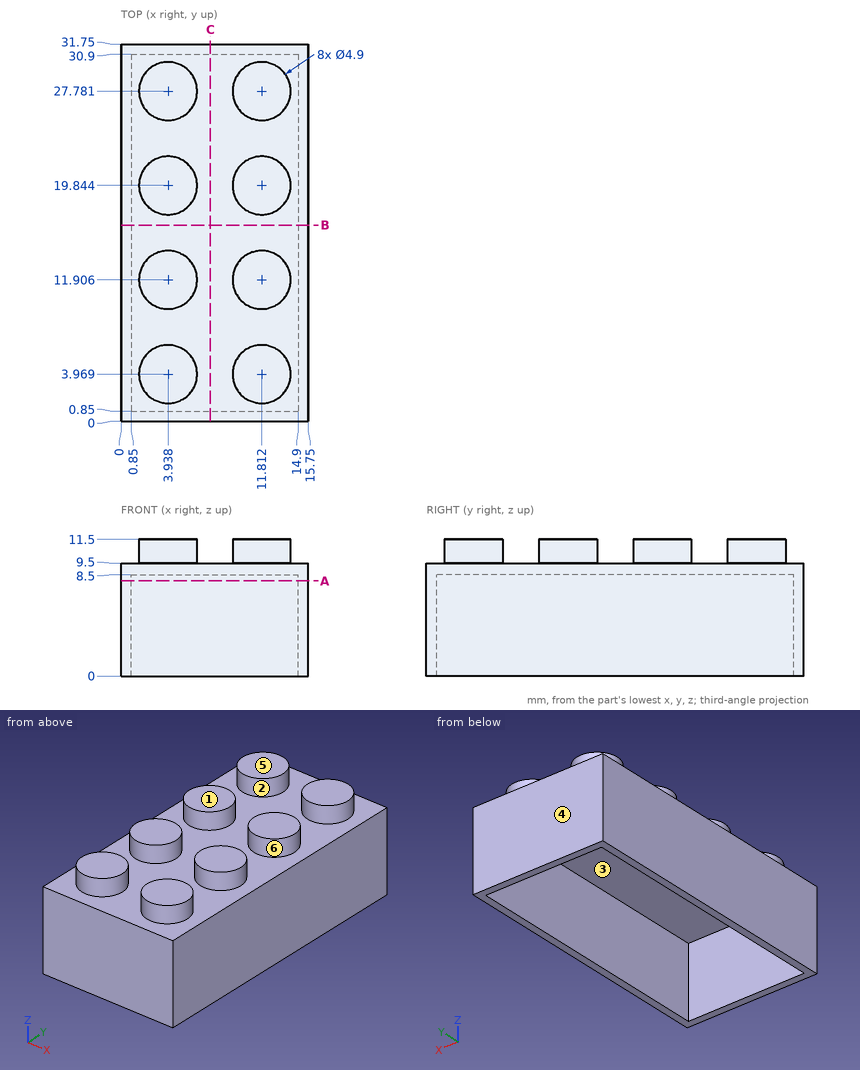
Source: three-view drawing plus pictorial views. Frame: mm from the lowest corner of the part. A direction names the side the tool comes from. Round coordinates to 2 decimals unless told otherwise and drop trailing zeros. Loops run counter-clockwise (first coordinate to the right, second up) from the corner with the lowest first, then second, coordinate; pieces in that order, holes last.
Item 1: Line query: L1, parallel to X at y = 12, z = 3.25; L2, parallel to Y at x = 6.75, z = 2.75; L3, parallel to Z at x = 7.5, y = 8. Output: solid intervals per line, ascending.
Checked values:
L1: x = 0 to 0.85, 14.9 to 15.75
L2: y = 0 to 0.85, 30.9 to 31.75
L3: z = 8.5 to 9.5
Item 2: Mould query, pull axis Y, two halves, no side actions, for the marked faces 4, 5 and 6. Classes: released by +Y, released by -Y, zero draft, split by the parting line, or undercut.
Checked values:
face 4: released by +Y
face 5: zero draft
face 6: undercut
Item 3: Reachability of the marked faces 1, 2 and 3 from +Z, -Z, +X, -X, +Y, -Y: full face, straight path, thin tool, end or side. Return the list, or none.
Checked values:
face 1: +Z, +X, -X, +Y, -Y
face 2: +Z
face 3: -Z
Item 4: Contact query for a flat-ended pin moving along its axis: P1, Ø3, axis at x = 10, y = 14, coming from the -Z side. Output: stop coordinate, or through.
Checked values:
P1: stops at z = 8.5
Item 5: Section C-C, the plane x = 7.5. Output: boundary loops of the cut face in (y, z).
Checked values:
outline: (0, 0) - (0.85, 0) - (0.85, 8.5) - (30.9, 8.5) - (30.9, 0) - (31.75, 0) - (31.75, 9.5) - (0, 9.5) - close
Item 6: Section A-A, the plane z = 8. Output: boundary loops of the cut face in (x, y).
Checked values:
outline: (0, 0) - (15.75, 0) - (15.75, 31.75) - (0, 31.75) - close; hole (0.85, 0.85) - (14.9, 0.85) - (14.9, 30.9) - (0.85, 30.9) - close
Item 7: Section B-B, the plane y = 16.5. Output: boundary loops of the cut face in (x, z).
Checked values:
outline: (0, 0) - (0.85, 0) - (0.85, 8.5) - (14.9, 8.5) - (14.9, 0) - (15.75, 0) - (15.75, 9.5) - (0, 9.5) - close
